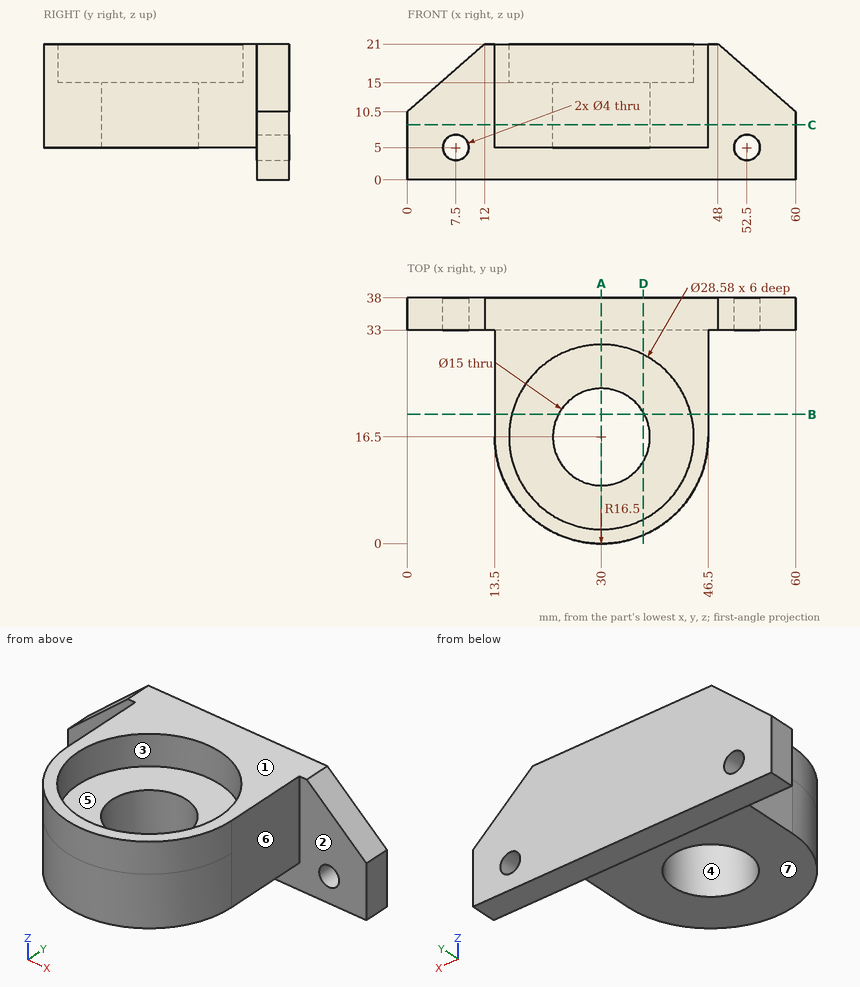
The figure shows three views and two pictorial views of one solid part (mm, origin at its lowest corner). Answer the questions. A direction names the side the tool comes from. Give positions to 0.01 mm unless a question says otherwise; leave off trailing zeros. Write each loop counter-clockwise with the first axis right and the second up, starting at its lowest first coordinate (ties: lowest second). Pieces come first, ordered by that corner, then holes. Notation, with made-up numbers: M -8.75,30 L 30.25,30 A15 ccw 30.25,39 Z; hole C 80,55.5 d6. An arc over 180 degrees is marked long. One line per item, written item: value. Start each with the question number.
(1) Find section D-D (x = 36.5). Determine the outline of the cut face in (y, z), plus the area to 3 significant figures.
(2) Find the intervals of material crossed by line 1 (X direction, y = 35.8, z = 5); line 2 (Y direction, x = 30, z = 11.5); line 3 (Z direction, x = 38.5, y = 31), in increasing order.
(3) Find section C-C (z = 8.5). Determine the outline of the cut face in (x, y), plus the area to 3 significant figures.
(4) Find section A-A (x = 30). Determine the outline of the cut face in (y, z), plus the area to 3 significant figures.
(5) Determine the mould class of the marked faces 1, 2, 3 and 4 for opening direction Y: pulls with the +Y half, pulls with the -Y half, needs draft (parallel to the pull), parting line crosses it, or undercut.
(6) Flat-ended cylindrical pins translate along their axes: pin 1 Ø5 at (x, z) = (7.5, 5) entering from -Y; pin 2 Ø6.5 at (x, z) = (22, 7.5) entering from -Y; pin 3 Ø10 at (y, z) = (19.5, 15) entering from +X; pin 4 Ø6 at (x, y) = (11.5, 25.5) entering from +Z. Find the tip coordinate at first contact, or state that the pin passes through.
(7) A tool of negligible diameter and unlimited length cuts with its end or side. For the marked faces 5, 6 and 7, from which of +Z, -Z, +X, -X, +Y, -Y can it reach the whole face along a straight path? Write none if from no direction.
(8) Find section B-B (y = 20). Determine the outline of the cut face in (x, z).
Results below:
1. outline: M 1.33,5 L 12.76,5 L 12.76,15 L 3.77,15 L 3.77,21 L 1.33,21 Z; M 20.24,5 L 33,5 L 33,0 L 38,0 L 38,21 L 29.23,21 L 29.23,15 L 20.24,15 Z
1. area: 384 mm^2
2. line 1: x = 0 to 5.5, 9.5 to 50.5, 54.5 to 60
2. line 2: y = 0 to 9, 24 to 38
2. line 3: z = 5 to 21
3. outline: M 0,33 L 13.5,33 L 13.5,16.5 A16.5 ccw 46.5,16.5 L 46.5,33 L 60,33 L 60,38 L 0,38 Z; hole C 30,16.5 d15
3. area: 1,100 mm^2
4. outline: M 0,5 L 9,5 L 9,15 L 2.21,15 L 2.21,21 L 0,21 Z; M 24,5 L 33,5 L 33,0 L 38,0 L 38,21 L 30.79,21 L 30.79,15 L 24,15 Z
4. area: 312 mm^2
5. face 1: needs draft
5. face 2: pulls with the -Y half
5. face 3: undercut
5. face 4: undercut
6. pin 1: stops at y = 33
6. pin 2: stops at y = 0.7
6. pin 3: stops at x = 46.5
6. pin 4: stops at z = 21
7. face 5: +Z
7. face 6: +Z, -Z, +X, -Y
7. face 7: -Z, +X, -X, -Y
8. outline: M 13.5,5 L 23.37,5 L 23.37,15 L 16.15,15 L 16.15,21 L 13.5,21 Z; M 36.63,5 L 46.5,5 L 46.5,21 L 43.85,21 L 43.85,15 L 36.63,15 Z
